Input: part model. Units: mm. Frame: model coordinates. Coordinates: 2 decimals unless noted, no trailing zeros. Write each loop counter-clockwise with the first axis right and the second up, starting at its lowest first coordinate (ties: lowest second). Pieces come first, ordered by that corner, then holes.
1) Section query A-A (y = -58). Output: boundary loops of the cut face in (x, z).
2) Section query B-B (x = -85). Output: boundary loops of the cut face in (y, z).
3) Line query: L1, parallel to X at y = -51.5, z = 0.7; L2, parallel to Y at x = -40.5, z = 0.55; L3, parallel to Y at x = -85, z = 1. Output: solid intervals per line, ascending.
4) Section query C-C (x = -6.5). Output: boundary loops of the cut face in (y, z), then the cut area to 3 significant figures.
5) Pin query (flat end, axial travel): pin 1 Ø3.5 at (x, y) = (77.5, -30.5) entering from -Z; pin 2 Ø12 at (x, y) = (-42, 20) entering from +Z. Return the tip coordinate at first contact, or that it passes through.
6) Section query D-D (z = 1.6). State how many separate pieces and enclosed holes the cut face has, then the cut area to 3 significant figures.
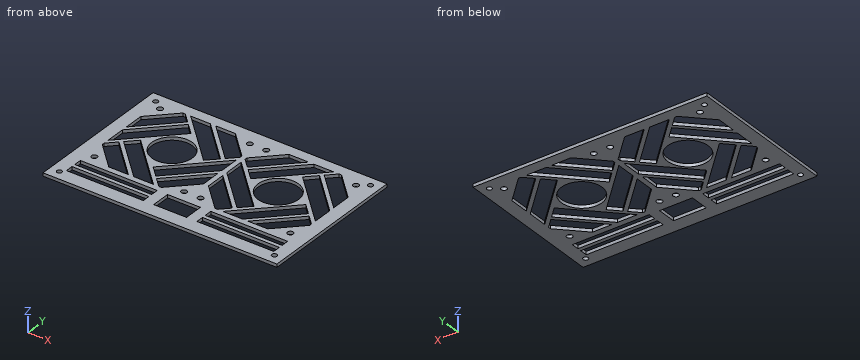
from build123d import *

# Parameters (mm, degrees)
SKETCH1_W               = 185
SKETCH1_H               = 115
BOSS_EXTRUDE1_DEPTH     = 2.5
SKETCH2_R               = 16
CUT_EXTRUDE1_DEPTH      = 114.369969569
SKETCH5_W               = 26
SKETCH5_H               = 15
CUT_EXTRUDE4_DEPTH      = 10
CUT_EXTRUDE7_DEPTH      = 10
SKETCH9_W               = 60.811183182
SKETCH9_H               = 6
CUT_EXTRUDE8_DEPTH      = 10
CUT_EXTRUDE9_DEPTH      = 114.369969569
CUT_EXTRUDE9_DEPTH_BACK = 114.369969569
SKETCH10_R              = 2.25
SKETCH11_R              = 2
CUT_EXTRUDE11_DEPTH     = 114.369969569
SKETCH12_W              = 185
SKETCH12_H              = 4
BOSS_EXTRUDE2_DEPTH     = 2.5


with BuildPart() as part:
    # Sketch1 → Boss-Extrude1 (new body)
    with BuildSketch(Plane.XY):
        with Locations((0, -8)):
            Rectangle(SKETCH1_W, SKETCH1_H)
    extrude(amount=BOSS_EXTRUDE1_DEPTH)

    # Sketch2 → Cut-Extrude1 (cut, through all)
    with BuildSketch(Plane.XY.offset(2.5)):
        with Locations((-42, 5)):
            Circle(SKETCH2_R)
        with Locations((42, 5)):
            Circle(SKETCH2_R)
    extrude(amount=-CUT_EXTRUDE1_DEPTH, mode=Mode.SUBTRACT)

    # Sketch5 → Cut-Extrude4 (cut)
    with BuildSketch(Plane.XY.offset(2.5)):
        with Locations((0, -47)):
            Rectangle(SKETCH5_W, SKETCH5_H)
    extrude(amount=-CUT_EXTRUDE4_DEPTH, mode=Mode.SUBTRACT)

    # Sketch8 → Cut-Extrude7 (cut)
    with BuildSketch(Plane.XY.offset(2.5)):
        Polygon((-82, 10.254833996), (-54.02081528, 38.234018716), (-60.786796564, 45), (-62.811183182, 45), (-82, 25.811183182), align=None)
        Polygon((-82, 6.012193309), (-51.899494937, 36.112698372), (-44.121320344, 28.334523779), (-82, -9.544155877), align=None)
        Polygon((-21.188816818, -35), (-2, -15.811183182), (-2, -0.254833996), (-29.97918472, -28.234018716), (-23.213203436, -35), align=None)
        Polygon((-43.012193309, -35), (-73.112698372, -4.899494937), (-65.334523779, 2.878679656), (-27.455844123, -35), align=None)
        Polygon((-82, -13.786796564), (-75.234018716, -7.02081528), (-47.254833996, -35), (-62.811183182, -35), (-82, -15.811183182), align=None)
        Polygon((-18.665476221, 7.121320344), (-56.544155877, 45), (-40.987806691, 45), (-10.887301628, 14.899494937), align=None)
        Polygon((-2, 25.811183182), (-21.188816818, 45), (-36.745166004, 45), (-8.765981284, 17.02081528), (-2, 23.786796564), align=None)
        Polygon((-2, 3.987806691), (-2, 19.544155877), (-39.878679656, -18.334523779), (-32.100505063, -26.112698372), align=None)
        Polygon((39.878679656, -18.334523779), (2, 19.544155877), (2, 3.987806691), (32.100505063, -26.112698372), align=None)
        Polygon((29.97918472, -28.234018716), (23.213203436, -35), (21.188816818, -35), (2, -15.811183182), (2, -0.254833996), align=None)
        Polygon((54.02081528, 38.234018716), (60.786796564, 45), (62.811183182, 45), (82, 25.811183182), (82, 10.254833996), align=None)
        Polygon((2, 23.786796564), (2, 25.811183182), (21.188816818, 45), (36.745166004, 45), (8.765981284, 17.02081528), align=None)
        Polygon((56.544155877, 45), (40.987806691, 45), (10.887301628, 14.899494937), (18.665476221, 7.121320344), align=None)
        Polygon((44.121320344, 28.334523779), (51.899494937, 36.112698372), (82, 6.012193309), (82, -9.544155877), align=None)
        Polygon((62.811183182, -35), (82, -15.811183182), (82, -13.786796564), (75.234018716, -7.02081528), (47.254833996, -35), align=None)
        Polygon((43.012193309, -35), (27.455844123, -35), (65.334523779, 2.878679656), (73.112698372, -4.899494937), align=None)
    extrude(amount=-CUT_EXTRUDE7_DEPTH, mode=Mode.SUBTRACT)

    # Sketch9 → Cut-Extrude8 (cut)
    with BuildSketch(Plane.XY.offset(2.5)):
        with Locations((-51.594408409, -42.5)):
            Rectangle(SKETCH9_W, SKETCH9_H)
        with Locations((51.594408409, -42.5)):
            Rectangle(SKETCH9_W, SKETCH9_H)
        with Locations((-51.594408409, -51.5)):
            Rectangle(SKETCH9_W, SKETCH9_H)
        with Locations((51.594408409, -51.5)):
            Rectangle(SKETCH9_W, SKETCH9_H)
    extrude(amount=-CUT_EXTRUDE8_DEPTH, mode=Mode.SUBTRACT)

    # Sketch10 → Cut-Extrude9 (cut, two sides: drawn at the far end of the back side and taken through both)
    with BuildSketch(Plane.XY.offset(2.5).offset(-CUT_EXTRUDE9_DEPTH_BACK)):
        with Locations((-77.5, 40.5)):
            Circle(SKETCH10_R)
        with Locations((-6.5, 40.5)):
            Circle(SKETCH10_R)
        with Locations((-6.5, -30.5)):
            Circle(SKETCH10_R)
        with Locations((-77.5, -30.5)):
            Circle(SKETCH10_R)
        with Locations(Location((77.5, -30.5, 0), (0, 0, 180))):
            Circle(SKETCH10_R)
        with Locations(Location((6.5, -30.5, 0), (0, 0, 180))):
            Circle(SKETCH10_R)
        with Locations(Location((6.5, 40.5, 0), (0, 0, 180))):
            Circle(SKETCH10_R)
        with Locations(Location((77.5, 40.5, 0), (0, 0, 180))):
            Circle(SKETCH10_R)
    extrude(amount=CUT_EXTRUDE9_DEPTH + CUT_EXTRUDE9_DEPTH_BACK, mode=Mode.SUBTRACT)

    # Sketch11 → Cut-Extrude11 (cut, through all)
    with BuildSketch(Plane.XY.offset(2.5)):
        with Locations((-85, 46)):
            Circle(SKETCH11_R)
        with Locations((85, 46)):
            Circle(SKETCH11_R)
        with Locations((85, -58)):
            Circle(SKETCH11_R)
        with Locations((-85, -58)):
            Circle(SKETCH11_R)
    extrude(amount=-CUT_EXTRUDE11_DEPTH, mode=Mode.SUBTRACT)

    # Sketch12 → Boss-Extrude2 (add)
    with BuildSketch(Plane.XY.offset(2.5)):
        with Locations((0, 51.5)):
            Rectangle(SKETCH12_W, SKETCH12_H)
    extrude(amount=-BOSS_EXTRUDE2_DEPTH)


solid = part.part
Answer:
1. outline: (-92.5, 0) - (-87, 0) - (-87, 2.5) - (-92.5, 2.5) - close; (-83, 0) - (83, 0) - (83, 2.5) - (-83, 2.5) - close; (87, 0) - (92.5, 0) - (92.5, 2.5) - (87, 2.5) - close
2. outline: (-65.5, 0) - (-60, 0) - (-60, 2.5) - (-65.5, 2.5) - close; (-56, 0) - (44, 0) - (44, 2.5) - (-56, 2.5) - close; (48, 0) - (53.5, 0) - (53.5, 2.5) - (48, 2.5) - close
3. L1: x = -92.5 to -82, -21.19 to -13, 13 to 21.19, 82 to 92.5
3. L2: y = -65.5 to -54.5, -48.5 to -45.5, -39.5 to -35, -21.96 to -10.93, 20.93 to 28.96, 44.51 to 53.5
3. L3: y = -65.5 to -60, -56 to 44, 48 to 53.5
4. outline: (-65.5, 0) - (-54.5, 0) - (-54.5, 2.5) - (-65.5, 2.5) - close; (-39.5, 0) - (-32.75, 0) - (-32.75, 2.5) - (-39.5, 2.5) - close; (-28.25, 0) - (-20.31, 0) - (-20.31, 2.5) - (-28.25, 2.5) - close; (-4.75, 0) - (-0.51, 0) - (-0.51, 2.5) - (-4.75, 2.5) - close; (15.04, 0) - (19.29, 0) - (19.29, 2.5) - (15.04, 2.5) - close; (30.31, 0) - (38.25, 0) - (38.25, 2.5) - (30.31, 2.5) - close; (42.75, 0) - (53.5, 0) - (53.5, 2.5) - (42.75, 2.5) - close
4. area: 132 mm2
5. pin 1: passes through
5. pin 2: stops at z = 2.5
6. separate pieces: 1
6. enclosed holes: 35
6. area: 11,200 mm2
